Verification items for the finished model (mm, model axes). Give positions to 0.01 mm unless a question says otherwise; leave off trailing zeros. Write each loop counter-clockwise with the first axis right and the second up, starting at its lowest first coordinate (ties: lowest second). Pieces come first, ordered by that corner, then holes. Notation, with made-up numbers: M 84,8.5 L 140,8.5 A23 ccw 140,47.5 Z; hole C -32,4 d7. An arc over 180 degrees is marked long. Write item = value, one per line.
from build123d import *

# Parameters (mm, degrees)
SKETCH7_R           = 1.3716
BOSS_EXTRUDE4_DEPTH = 4.7498


with BuildPart() as part:
    # Sketch7 → Boss-Extrude4 (new, symmetric)
    with BuildSketch(Plane.XY):
        Polygon((-76.439762625, 4.738534743), (-76.86239804, 8.282120356), (-80.142550908, 9.687900156), (-83.000068362, 7.550094344), (-82.577432948, 4.006508731), (-79.297280079, 2.600728931), align=None)
        with Locations((-79.719915494, 6.144314544)):
            Circle(SKETCH7_R, mode=Mode.SUBTRACT)
    extrude(amount=BOSS_EXTRUDE4_DEPTH, both=True)


solid = part.part
1) Cross-section at C-C on y = 5. Record the boundary of the cut face in (x, z).
From the geometry:
outline = M -82.7,-4.75 L -80.48,-4.75 L -80.48,4.75 L -82.7,4.75 Z; M -78.96,-4.75 L -76.47,-4.75 L -76.47,4.75 L -78.96,4.75 Z
2) Cross-section at B-B on z = -2. Record the boundary of the cut face in (x, y).
From the geometry:
outline = M -83,7.55 L -82.58,4.01 L -79.3,2.6 L -76.44,4.74 L -76.86,8.28 L -80.14,9.69 Z; hole C -79.72,6.14 d2.74
3) Draft check along Y on faces 1 (the cylindrical face through (-78.453, 5.619, -0.066)), 2 (the flat face through (-76.65, 6.49, 0.07)), 3 (the flat face through (-77.889, 3.655, 0.066)). Enter one of: +Y half, -Y half, draft (parallel to the pull), parting line (faces both ways), or undercut.
From the geometry:
face_1 = undercut
face_2 = +Y half
face_3 = -Y half
4) Depth check by flat-ended pin: P1, Ø4, axis at y = 8.5, z = -1, coming from the -X side; P2, Ø1.5, axis at y = 4, z = 3, coming from the -X side; P3, Ø1, axis at x = -80.5, z = -3.5, coming from the -Y side; P4, Ø2, axis at x = -79.5, z = -1.5, coming from the -Y side. Enter the tip coordinate at first touch or a pass-through.
From the geometry:
P1 = -83
P2 = -82.67
P3 = 2.9
P4 = 2.6
5) Material ranges on probe 1 along Y at (x, z) = (-79, -0.5); probe 2 along X at (y, z) = (6.5, 0); probe 3 along Y at (x, z) = (-80.25, 2), recorded low to high. Write a range as from..to.
From the geometry:
probe_1 = 2.82..4.98, 7.31..9.2
probe_2 = -82.87..-81.04, -78.4..-76.65
probe_3 = 3.01..4.88, 7.41..9.61
6) Cross-section at D-D on x = -77. Record the boundary of the cut face in (y, z).
From the geometry:
outline = M 4.32,-4.75 L 8.34,-4.75 L 8.34,4.75 L 4.32,4.75 Z
7) Cross-section at A-A on x = -79. Record the boundary of the cut face in (y, z).
From the geometry:
outline = M 2.82,-4.75 L 4.98,-4.75 L 4.98,4.75 L 2.82,4.75 Z; M 7.31,-4.75 L 9.2,-4.75 L 9.2,4.75 L 7.31,4.75 Z
